For this review, take the finished solid that the model builds, in its own axes (mm). A direction names the side the tool comes from. Round coordinates to 2 decimals unless told otherwise and drop trailing zeros. Loops run counter-clockwise (first coordinate to the right, second up) from the corner with the lowest first, then second, coordinate; pieces in that order, holes last. Notation, with made-up numbers: (-14.5, 80) -> (-10.5, 80) arc R18 ccw to (-10.5, 91) -> close; hole circle Ø1 at (81.5, 24.5). An arc over 180 degrees is marked (long way). Write each question's results on one line, items separated by ' | '.
```python
from build123d import *

# Parameters (mm, degrees)
F0_W     = 35.4
F0_H     = 7
F1_DEPTH = 3
F2_W     = 1.8
F2_H     = 1
F3_DEPTH = 0.6
F4_R     = 1
F5_DEPTH = 0.1
F7_DEPTH = 0.5


with BuildPart() as f1:
    # F0 (on Top) → F1 (new body)
    with BuildSketch(Plane.XY):
        with Locations((17.7, 3.5)):
            Rectangle(F0_W, F0_H)
    extrude(amount=F1_DEPTH)

    # F2 (on face) → F3 (cut)
    with BuildSketch(Plane(origin=(0, 0, 0), x_dir=(1, 0, 0), z_dir=(0, 0, -1))):
        with Locations((1.19, -0.5)):
            Rectangle(F2_W, F2_H)
        with Locations((3.73, -0.5)):
            Rectangle(F2_W, F2_H)
        with Locations((6.27, -0.5)):
            Rectangle(F2_W, F2_H)
        with Locations((8.81, -0.5)):
            Rectangle(F2_W, F2_H)
        with Locations((11.35, -0.5)):
            Rectangle(F2_W, F2_H)
        with Locations((13.89, -0.5)):
            Rectangle(F2_W, F2_H)
        with Locations((16.43, -0.5)):
            Rectangle(F2_W, F2_H)
        with Locations((18.97, -0.5)):
            Rectangle(F2_W, F2_H)
        with Locations((21.51, -0.5)):
            Rectangle(F2_W, F2_H)
        with Locations((24.05, -0.5)):
            Rectangle(F2_W, F2_H)
        with Locations((26.59, -0.5)):
            Rectangle(F2_W, F2_H)
        with Locations((29.13, -0.5)):
            Rectangle(F2_W, F2_H)
        with Locations((31.67, -0.5)):
            Rectangle(F2_W, F2_H)
        with Locations((34.21, -0.5)):
            Rectangle(F2_W, F2_H)
        with Locations((34.21, -6.5)):
            Rectangle(F2_W, F2_H)
        with Locations((31.67, -6.5)):
            Rectangle(F2_W, F2_H)
        with Locations((29.13, -6.5)):
            Rectangle(F2_W, F2_H)
        with Locations((26.59, -6.5)):
            Rectangle(F2_W, F2_H)
        with Locations((24.05, -6.5)):
            Rectangle(F2_W, F2_H)
        with Locations((21.51, -6.5)):
            Rectangle(F2_W, F2_H)
        with Locations((18.97, -6.5)):
            Rectangle(F2_W, F2_H)
        with Locations((16.43, -6.5)):
            Rectangle(F2_W, F2_H)
        with Locations((13.89, -6.5)):
            Rectangle(F2_W, F2_H)
        with Locations((11.35, -6.5)):
            Rectangle(F2_W, F2_H)
        with Locations((8.81, -6.5)):
            Rectangle(F2_W, F2_H)
        with Locations((6.27, -6.5)):
            Rectangle(F2_W, F2_H)
        with Locations((3.73, -6.5)):
            Rectangle(F2_W, F2_H)
        with Locations((1.19, -6.5)):
            Rectangle(F2_W, F2_H)
    extrude(amount=-F3_DEPTH, mode=Mode.SUBTRACT)

    # F4 (on face) → F5 (cut)
    with BuildSketch(Plane.XY.offset(3)):
        with Locations((5.08, 3.5)):
            Circle(F4_R)
        with Locations((30.32, 3.5)):
            Circle(F4_R)
    extrude(amount=-F5_DEPTH, mode=Mode.SUBTRACT)

    # F6 (on face) → F7 (cut)
    with BuildSketch(Plane.XY.offset(3)):
        with BuildLine():
            Line((0, 4.25), (0, 2.75))
            ThreePointArc((0, 2.75), (0.75, 3.5), (0, 4.25))
        make_face()
    extrude(amount=-F7_DEPTH, mode=Mode.SUBTRACT)


solid = f1.part
```
1. To check wall thickness, follow probe 1 along Z at (x, y) = (23.5, 0.75). State the ranges of the line that lie inside material, in increasing order.
Values found:
probe 1: z = 0.6 to 3
2. Draft analysis for pull direction X (two halves, no side actions). For faces 4 (the face through (1.2, 6.5, 0.6)), 5 (the face through (0, 3, 1)), state which applies: released by +X, released by -X, zero draft, split by the parting line, or undercut.
Values found:
face 4: undercut | face 5: released by -X
3. Tool access review of faces 1 (the face through (26.6, 0.5, 0.6)), 2 (the face through (11.3, 6.5, 0.6)), 3 (the face through (5, 4, 2.9)): name each direction out of +Z, -Z, +X, -X, +Y, -Y from which nothing blocks a thin tool from reaching the whole face with its end or side.
Values found:
face 1: -Z, -Y | face 2: -Z, +Y | face 3: +Z
4. Consider section A-A (x = 21). State the section outline as (y, z) points.
Values found:
outline: (0, 0.6) -> (1, 0.6) -> (1, 0) -> (6, 0) -> (6, 0.6) -> (7, 0.6) -> (7, 3) -> (0, 3) -> close
5. For pin 1 (0.5 mm diameter, centred on y = 0.5, z = 0.5, fed in from -X), flat-tipped, find the tip position at first contact; note if it passes through.
Values found:
pin 1: stops at x = 0
